Input: part model. Units: mm. Frame: model coordinates. A direction names the side the tool comes from. Coordinates: 2 decimals unless noted, no trailing zeros. Loops run counter-clockwise (first coordinate to the right, second up) from the corner with the lowest first, then second, coordinate; pieces in that order, holes last.
Item 1: Reachability of faces 1 (the flat face through (0, -4, -4)), 2 (the cylindrical face through (16.703, 8.767, -16.856)) from +Z, -Z, +X, -X, +Y, -Y: full face, straight path, thin tool, end or side. Return the list, or none.
Item 2: Ray query, line 1 along Z through (x, y) = (9, 0); line 2 along Y through (x, z) = (17, -5.5); line 3 along Y through (x, z) = (28.5, -6.5). Return the intervals inside material, ascending.
Item 3: Section C-C on x = 32. Return loops of the section in (y, z), and give its area (3 significant figures).
Item 4: Pull-direction query (Y, two-part tool) for faces 3 (the flat face through (40, 10, -11.5)), 4 (the conical face through (0.13, 8.27, -15.9)), 5 (the flat face through (12, 0, -6)), 6 (the cylindrical face through (5.9, 2.4, -4.5)); classes: released by +Y, released by -Y, zero draft, split by the parting line, or undercut.
Item 5: Contact query for flat-ended pins moving along their axis: P1, Ø2, axis at x = 19, y = -3, coming from the +Z side; P2, Ø1.5, axis at x = 23, y = 13.5, coming from the +Z side; P3, Ø8, axis at x = 22, y = 8, coming from the +Z side. Output: stop coordinate, or through.
Item 6: Section A-A on y = 0. Return loops of the section in (x, z), and give its area (3 significant figures).
```python
from build123d import *


with BuildPart() as part:
    # Sketch1 → Revolve1 (revolve)
    with BuildSketch(Plane.XY):
        with BuildLine():
            Line((0, 17.845299462), (2, 19))
            Line((2, 19), (31, 19))
            Line((31, 19), (31, 22.5))
            Line((31, 22.5), (37, 22.5))
            ThreePointArc((37, 22.5), (39.121320344, 21.621320344), (40, 19.5))
            Line((40, 19.5), (40, 15))
            Line((40, 15), (12.772080403, 14.049180096))
            ThreePointArc((12.772080403, 14.049180096), (12.22452816, 13.805394131), (12, 13.249667434))
            Line((12, 13.249667434), (12, 5.1))
            Line((12, 5.1), (0, 5.1))
            Line((0, 5.1), (0, 17.845299462))
        make_face()
    revolve(axis=Axis((0, 0, 0), (1, 0, 0)))


solid = part.part
```
Results found:
1. face 1: +Z, -Z, -X, +Y, -Y
1. face 2: -X
2. line 1: z = -19 to -5.1, 5.1 to 19
2. line 2: y = -18.19 to -13.09, 13.09 to 18.19
2. line 3: y = -17.85 to -13.07, 13.07 to 17.85
3. outline: circle Ø45 at (0, 0); hole circle Ø29.44 at (0, 0)
3. area: 910 mm2
4. face 3: zero draft
4. face 4: split by the parting line
4. face 5: undercut
4. face 6: undercut
5. P1: stops at z = 18.89
5. P2: stops at z = 14.09
5. P3: stops at z = 18.57
6. outline: (0, -17.85) - (2, -19) - (31, -19) - (31, -22.5) - (37, -22.5) arc R3 ccw to (40, -19.5) - (40, -15) - (12.77, -14.05) arc R0.8 cw to (12, -13.25) - (12, -5.1) - (0, -5.1) - close; (0, 5.1) - (12, 5.1) - (12, 13.25) arc R0.8 cw to (12.77, 14.05) - (40, 15) - (40, 19.5) arc R3 ccw to (37, 22.5) - (31, 22.5) - (31, 19) - (2, 19) - (0, 17.85) - close
6. area: 642 mm2
